```python
from build123d import *

# Parameters (mm, degrees)
F1_DEPTH = 76.2
F4_D     = 4.318
F4_DEPTH = 12.7
F4_TIP   = 1.2972580765
F5_R     = 3.96875
F5_R_2   = 2.159
F6_DEPTH = 2.54


with BuildPart() as f1:
    # F0 (on Front) → F1 (new body)
    with BuildSketch(Plane.XZ):
        Polygon((0, 63.5), (0, 0), (9.525, 0), (9.525, 10.16), (6.985, 12.7), (6.985, 22.86), (9.525, 25.4), (9.525, 38.1), (6.985, 40.64), (6.985, 50.8), (9.525, 53.34), (9.525, 63.5), align=None)
    extrude(amount=F1_DEPTH)

    # F4
    with Locations(Plane.YZ.offset(9.525)):
        with Locations((-63.5, 58.42), (-12.7, 58.42), (-63.5, 5.08), (-12.7, 5.08)):
            Hole(F4_D / 2, depth=F4_DEPTH)
            with Locations((0, 0, -(F4_DEPTH + F4_TIP / 2))):  # 118° drill point
                Cone(0, F4_D / 2, F4_TIP, mode=Mode.SUBTRACT)

    # F5 (on face) → F6 (cut)
    with BuildSketch(Plane.YZ.offset(9.525)):
        with Locations((-63.5, 58.42)):
            Circle(F5_R)
        with Locations((-12.7, 58.42)):
            Circle(F5_R)
        with Locations((-63.5, 5.08)):
            Circle(F5_R)
        with Locations((-63.5, 5.08)):
            Circle(F5_R_2, mode=Mode.SUBTRACT)
        with Locations((-12.7, 5.08)):
            Circle(F5_R)
        with Locations((-12.7, 5.08)):
            Circle(F5_R_2, mode=Mode.SUBTRACT)
    extrude(amount=-F6_DEPTH, mode=Mode.SUBTRACT)


solid = f1.part
```
Geometry: final body of the model. Coordinates: model frame, mm. A direction names the side the tool comes from. Round coordinates to 2 decimals unless told otherwise and drop trailing zeros. Order: outer loops, then holes, each group sorted by start corner. A loop starts at its lowest first (then second) coordinate and runs counter-clockwise, first axis right, second up. Notation, with made-up numbers: (73, 87.5) - (92, 87.5) arc R23 ccw to (92, 122.5) - close; hole circle Ø11 at (64.5, 68.25). An arc over 180 degrees is marked (long way). Write item = value, one per line. Start each with the question number.
Q1. Pull-direction query (Y, two-part tool) for faces 4 (the flat face through (8.273, -37.567, 39.352)), 5 (the flat face through (5, 0, 32)), 6 (the cylindrical face through (3.444, -64.496, 56.505)); classes: +Y half, -Y half, draft (parallel to the pull), parting line (faces both ways), or undercut.
Q2. Pin query (flat end, axial travel): pin 1 (5.5 mm diameter, centred on y = -63.5, z = 58.42, fed in from +X) (3 decimals); pin 2 (12.5 mm diameter, centred on y = -12.7, z = 58.42, fed in from -X); pin 3 (11 mm diameter, centred on y = -48, z = 18, fed in from +X) (3 decimals). Return the tip coordinate at first contact, or that it passes through.
Q3. Cut plane D-D on y = -27. Return the cut outline in (x, z) (3 decimals), and give its area (3 significant figures).
Q4. Cut plane A-A on y = -12.7. Return the cut outline in (x, z) (3 decimals), and give its area (3 significant figures).
Q5. Access query for faces 1 (the flat face through (6.985, -38, 46)), 2 (the flat face through (5, -38, 0)), 3 (the cylindrical face through (8.273, -67.465, 5.254)). Directions: +Z, -Z, +X, -X, +Y, -Y. A direction counts if a zero-diameter tool reaches every point of the face in a straight line with its end or side. Return the directions, or none.
Q6. Ray query, line 1 (Y direction, x = 3.25, z = 5.08); line 2 (Z direction, x = 5.5, y = -63.5); line 3 (Z direction, x = 8.5, y = -11.5) (3 decimals). Return the intervals inside material, ascending. Write a range as from..to.
Q7. Cut plane B-B on z = 58.42. Return the cut outline in (x, y) (3 decimals).
Q8. Cut plane C-C on x = 8. Return the cut outline in (y, z) (1 decimal), and give its area (3 significant figures).
Outcome:
q1.face_4 = draft
q1.face_5 = +Y half
q1.face_6 = undercut
q2.pin_1 = 6.985
q2.pin_2 = 0
q2.pin_3 = 7.625
q3.outline = (0, 0) - (9.525, 0) - (9.525, 10.16) - (6.985, 12.7) - (6.985, 22.86) - (9.525, 25.4) - (9.525, 38.1) - (6.985, 40.64) - (6.985, 50.8) - (9.525, 53.34) - (9.525, 63.5) - (0, 63.5) - close
q3.area = 540 mm^2
q4.outline = (0, 0) - (9.525, 0) - (9.525, 1.111) - (6.985, 1.111) - (6.985, 2.921) - (0, 2.921) - close; (0, 7.239) - (6.985, 7.239) - (6.985, 9.049) - (9.525, 9.049) - (9.525, 10.16) - (6.985, 12.7) - (6.985, 22.86) - (9.525, 25.4) - (9.525, 38.1) - (6.985, 40.64) - (6.985, 50.8) - (9.525, 53.34) - (9.525, 54.451) - (6.985, 54.451) - (6.985, 56.261) - (0, 56.261) - close; (0, 60.579) - (6.985, 60.579) - (6.985, 62.389) - (9.525, 62.389) - (9.525, 63.5) - (0, 63.5) - close
q4.area = 440 mm^2
q5.face_1 = +X, +Y, -Y
q5.face_2 = -Z, +X, -X, +Y, -Y
q5.face_3 = +X
q6.line_1 = -76.2..-65.66, -61.34..-14.86, -10.54..0
q6.line_2 = 0..2.92, 7.24..56.26, 60.58..63.5
q6.line_3 = 0..1.297, 8.863..11.185, 24.375..39.125, 52.315..54.637, 62.203..63.5
q7.outline = (0, -76.2) - (9.525, -76.2) - (9.525, -67.469) - (6.985, -67.469) - (6.985, -65.659) - (0, -65.659) - close; (0, -61.341) - (6.985, -61.341) - (6.985, -59.531) - (9.525, -59.531) - (9.525, -16.669) - (6.985, -16.669) - (6.985, -14.859) - (0, -14.859) - close; (0, -10.541) - (6.985, -10.541) - (6.985, -8.731) - (9.525, -8.731) - (9.525, 0) - (0, 0) - close
q8.outline = (-76.2, 0) - (0, 0) - (0, 11.7) - (-76.2, 11.7) - close; (-76.2, 23.9) - (0, 23.9) - (0, 39.6) - (-76.2, 39.6) - close; (-76.2, 51.8) - (0, 51.8) - (0, 63.5) - (-76.2, 63.5) - close; hole circle Ø7.9 at (-63.5, 5.1); hole circle Ø7.9 at (-63.5, 58.4); hole circle Ø7.9 at (-12.7, 5.1); hole circle Ø7.9 at (-12.7, 58.4)
q8.area = 2,780 mm^2
